```python
from build123d import *

# Parameters (mm, degrees)
F0_R     = 2.667
F1_DEPTH = 5.588
F2_DEPTH = 5.588
F3_COUNT = 22
F5_R     = 6.35
F5_R_2   = 2.667
F6_DEPTH = 1.27
F4_R     = 5.969
F4_R_2   = 2.667
F7_DEPTH = 1.524


with BuildPart() as f1:
    # F0 (on Top) → F1 (new body)
    with BuildSketch(Plane.XY):
        with BuildLine():
            ThreePointArc((-0.7982498419, 7.705764478), (-5.1880616551, -5.753262141), (7.747, 0))
            ThreePointArc((7.747, 0), (5.5544090358, 5.4004212116), (0.2177501581, 7.74393917))
            ThreePointArc((0.2177501581, 7.74393917), (-0.2908767737, 7.7415372958), (-0.7982498419, 7.705764478))
        make_face()
        Circle(F0_R, mode=Mode.SUBTRACT)
    extrude(amount=F1_DEPTH)

    # F0 (on Top) → F2 (join)
    with BuildSketch(Plane.XY):
        with BuildLine():
            ThreePointArc((-0.7982498419, 7.705764478), (-0.2908767737, 7.7415372958), (0.2177501581, 7.74393917))
            Line((0.2177501581, 7.74393917), (0.2177501581, 8.6572673449))
            Line((0.2177501581, 8.6572673449), (0, 8.875017503))
            Line((0, 8.875017503), (-0.141982497, 9.017))
            Line((-0.141982497, 9.017), (-0.4385171868, 9.017))
            Line((-0.4385171868, 9.017), (-0.7194063476, 8.7361108392))
            Line((-0.7194063476, 8.7361108392), (-0.7982498419, 8.6572673449))
            Line((-0.7982498419, 8.6572673449), (-0.7982498419, 7.705764478))
        make_face()
    extrude(amount=F2_DEPTH)

    # F3: F1 ×22 about axis
    f3_axis = Axis((0, 0, 0), (0, 0, -1))


with BuildPart() as f1_1:
    add(f1.part)
    for i in range(1, F3_COUNT):
        add(f1.part.rotate(f3_axis, i * 360 / F3_COUNT))

    # F5 (on face) → F6 (cut)
    with BuildSketch(Plane.XY):
        Circle(F5_R)
        Circle(F5_R_2, mode=Mode.SUBTRACT)
    extrude(amount=F6_DEPTH, mode=Mode.SUBTRACT)

    # F4 (on face) → F7 (cut)
    with BuildSketch(Plane.XY.offset(5.588)):
        Circle(F4_R)
        Circle(F4_R_2, mode=Mode.SUBTRACT)
    extrude(amount=-F7_DEPTH, mode=Mode.SUBTRACT)


solid = f1_1.part
```
Input: part model. Units: mm. Frame: model coordinates. A direction names the side the tool comes from. Give positions to 0.01 mm unless a question says otherwise; leave off trailing zeros. One line per item, written item: value.
1. Line query: probe 1 along X at (y, z) = (7, 5.05); probe 2 along X at (y, z) = (8, 4.2); probe 3 along Z at (x, y) = (-2.25, -4.75). Output: solid intervals per line, ascending.
Determined:
probe 1: -5.32 to -4.24, -3.32 to 3.32, 3.55 to 4.76
probe 2: -3.18 to -2.12, -0.8 to 0.22, 1.52 to 2.58
probe 3: 1.27 to 4.06
2. Pin query (flat end, axial travel): pin 1 Ø10 at (x, y) = (1.5, -0.5) entering from -Z; pin 2 Ø6 at (x, y) = (0, 0) entering from -Z; pin 3 Ø1 at (y, z) = (3, 2.5) entering from -X; pin 4 Ø1 at (y, z) = (5.5, 3.5) entering from -X. Return the tip coordinate at first contact, or that it passes through.
Determined:
pin 1: z = 0
pin 2: z = 1.27
pin 3: x = -8.38
pin 4: x = -7.1
3. Reachability of faces 4 (the face through (-1.38, -6.2, 0.63)), 5 (the face through (8.08, -1.38, 2.75)), 6 (the face through (3, -1, 4.064)), 7 (the face through (-8.14, -0.95, 2.75)) from +Z, -Z, +X, -X, +Y, -Y: full face, straight path, thin tool, end or side. Return the list, or none.
Determined:
face 4: -Z
face 5: +Z, -Z
face 6: +Z
face 7: +Z, -Z, -X
4. Draft query along Y for faces 1 (the face through (-3.755, -7.32, 2.755)), 2 (the face through (0.822, 7.703, 2.755)), 3 (the face through (7.991, 1.955, 2.755)). Return one class per face: released by +Y, released by -Y, zero draft, split by the parting line, or undercut.
Determined:
face 1: released by -Y
face 2: released by +Y
face 3: undercut
